The listing builds one solid part. Answer for the finished solid, in the listing's coordinates (mm). A direction names the side the tool comes from. Coordinates: 2 decimals unless noted, no trailing zeros. Answer in a Markdown table with one row per item.
```python
from build123d import *

# Parameters (mm, degrees)
F0_W     = 127
F0_H     = 127
F1_DEPTH = 50.8
F2_W     = 20.632386
F2_H     = 12.723304
F2_W_2   = 12.7
F2_H_2   = 25.4
F2_W_3   = 19.256888
F2_H_3   = 11.347811
F2_W_4   = 15.130423
F2_W_5   = 19.944644
F2_H_4   = 12.723305
F3_DEPTH = 5.08


with BuildPart() as f1:
    # F0 (on Front) → F1 (new body)
    with BuildSketch(Plane.XZ):
        with Locations((-10.951542, 9.803599)):
            Rectangle(F0_W, F0_H)
    extrude(amount=F1_DEPTH)

    # F2 (on face) → F3 (cut)
    with BuildSketch(Plane(origin=(0, 0, -53.696401), x_dir=(1, 0, 0), z_dir=(0, 0, -1))):
        with Locations((-56.395188, 37.99798)):
            Rectangle(F2_W, F2_H)
        with Locations((-22.191468, 12.7)):
            Rectangle(F2_W_2, F2_H_2)
        with Locations((6.877462, 37.310233)):
            Rectangle(F2_W_3, F2_H_3)
        with Locations((41.264772, 37.310233)):
            Rectangle(F2_W_4, F2_H_3)
        with Locations((26.478228, 14.614607)):
            Rectangle(F2_W_5, F2_H_4)
    extrude(amount=-F3_DEPTH, mode=Mode.SUBTRACT)


solid = f1.part
```
(1) A flat-ended cylindrical pin translates along its axis: pin 1 (6.5 mm diameter, centred on x = -60.5, y = -38, fed in from -Z). Find the tip coordinate at first contact, or state that the pin passes through.
Check values:
| item | result |
|---|---|
| pin 1 | z = -48.62 |
(2) For a pull along X with two mould halves and no side action, classify faces 4 (the flat face through (52.548, -25, 9)), 5 (the flat face through (-12, -25, -53.696)), 6 (the flat face through (-57, -38, -48.616)) as released by +X, released by -X, zero draft, split by the parting line, or undercut.
Check values:
| item | result |
|---|---|
| face 4 | released by +X |
| face 5 | zero draft |
| face 6 | undercut |
(3) Which of the six approach directions +Z, -Z, +X, -X, +Y, -Y give full straight-line access (tool end or side, diameter ignored) to faces 1 (the flat face through (-22, -25.4, -51)), 2 (the flat face through (-74.452, -25, 9)), 3 (the flat face through (41, -31.636, -51))?
Check values:
| item | result |
|---|---|
| face 1 | -Z, +Y |
| face 2 | +Z, -Z, -X, +Y, -Y |
| face 3 | -Z |
(4) Find the intervals of material crossed by line 1 along Z through (x, y) = (-27.5, -12), in increasing order. Write a range as from..to.
Check values:
| item | result |
|---|---|
| line 1 | -48.62..73.3 |
